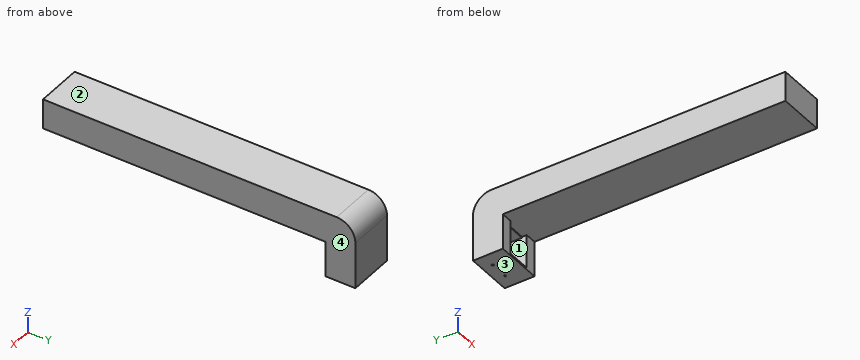
```python
from build123d import *

# Parameters (mm, degrees)
SKETCH_1_W          = 50
SKETCH_1_H          = 55
EXTRUDE_1_DEPTH     = 70
SKETCH_3_W          = 50
SKETCH_3_H          = 25
CUT_EXTRUDE_1_DEPTH = 38
SKETCH_4_W          = 25.5
SKETCH_4_H          = 36
CUT_EXTRUDE_2_DEPTH = 22
SKETCH_12_W         = 25.5
SKETCH_12_H         = 1
EXTRUDE_2_DEPTH     = 19
EXTRUDE_3_DEPTH     = 2
SKETCH_16_W         = 50
SKETCH_16_H         = 32
EXTRUDE_5_DEPTH     = 280
FILLET_1_R          = 20
SKETCH_23_R         = 1
CUT_EXTRUDE_3_DEPTH = 10


with BuildPart() as part:
    # 草图1 → 凸台-拉伸1 (new body)
    with BuildSketch(Plane.XY):
        with Locations((25, 27.5)):
            Rectangle(SKETCH_1_W, SKETCH_1_H)
    extrude(amount=EXTRUDE_1_DEPTH)

    # 草图3 → 切除-拉伸1 (cut)
    with BuildSketch(Plane(origin=(0, 0, 0), x_dir=(-1, 0, 0), z_dir=(0, 0, -1))):
        with Locations((-25, 12.5)):
            Rectangle(SKETCH_3_W, SKETCH_3_H)
    extrude(amount=-CUT_EXTRUDE_1_DEPTH, mode=Mode.SUBTRACT)

    # 草图4 → 切除-拉伸2 (cut)
    with BuildSketch(Plane.XZ.offset(-25)):
        with Locations((24.95, 20)):
            Rectangle(SKETCH_4_W, SKETCH_4_H)
    extrude(amount=-CUT_EXTRUDE_2_DEPTH, mode=Mode.SUBTRACT)

    # 草图12 → 凸台-拉伸2 (add)
    with BuildSketch(Plane.XZ.offset(-47)):
        with Locations((24.95, 37.5)):
            Rectangle(SKETCH_12_W, SKETCH_12_H)
    extrude(amount=EXTRUDE_2_DEPTH)

    # 草图13 → 凸台-拉伸3 (add)
    with BuildSketch(Plane.XZ.offset(-25)):
        Polygon((12.2, 38), (0, 38), (0, 0), (50, 0), (50, 38), (37.7, 38), (37.7, 2), (12.2, 2), align=None)
    extrude(amount=EXTRUDE_3_DEPTH)

    # 草图16 → 凸台-拉伸5 (add)
    with BuildSketch(Plane.XZ):
        with Locations((25, 54)):
            Rectangle(SKETCH_16_W, SKETCH_16_H)
    extrude(amount=EXTRUDE_5_DEPTH)

    # 圆角1
    fillet_1_edges = [part.edges().sort_by_distance(p)[0] for p in [
        (25, 55, 70),
    ]]
    fillet(fillet_1_edges, radius=FILLET_1_R)

    # 草图23 → 切除-拉伸3 (cut)
    with BuildSketch(Plane(origin=(0, 0, 0), x_dir=(-1, 0, 0), z_dir=(0, 0, -1))):
        with Locations((-15.2, 44.140200043)):
            Circle(SKETCH_23_R)
        with Locations((-34.8, 44.140200043)):
            Circle(SKETCH_23_R)
    extrude(amount=-CUT_EXTRUDE_3_DEPTH, mode=Mode.SUBTRACT)


solid = part.part
```
Could you check a few things on this model? Use its own coordinates, in mm. Face numbers are marked on the shaded views. Round coordinates to 2 decimals unless told otherwise and drop trailing zeros. Write each loop counter-clockwise with the first axis right and the second up, starting at its lowest first coordinate (ties: lowest second). Pieces come first, ordered by that corner, then holes.
(1) Thinking about a two-plate mould opening in Z: for the marked faces 1, 2, 3 and 4, which applies, +Z half, -Z half, draft (parallel to the pull), parting line (faces both ways), or undercut?
Findings below:
face 1: undercut
face 2: +Z half
face 3: -Z half
face 4: draft
(2) Suppose I cut it at D-D on x = 20.5. Write out the boundary of the cut face in (y, z).
Findings below:
outline: (-280, 38) - (28, 38) - (28, 37) - (47, 37) - (47, 2) - (23, 2) - (23, 0) - (55, 0) - (55, 50) arc R20 ccw to (35, 70) - (-280, 70) - close
(3) Suppose I cut it at A-A on z = 30.5. Write out the boundary of the cut face in (x, y).
Findings below:
outline: (0, 23) - (12.2, 23) - (12.2, 47) - (37.7, 47) - (37.7, 23) - (50, 23) - (50, 55) - (0, 55) - close
(4) For pin 1 (1.2 mm diameter, centred on x = 15.2, y = 44.14, fed in from -Z); pin 2 (8 mm diameter, centred on x = 40, y = -48, fed in from -Z); pin 3 (1 mm diameter, centred on x = 30.5, z = 13, fed in from -Y), each with a flat end and sliding along its axis, tell me the tip position at first contact or that it passes through.
Findings below:
pin 1: stops at z = 37
pin 2: stops at z = 38
pin 3: stops at y = 47
(5) Suppose I cut it at B-B on x = 7. Write out the boundary of the cut face in (y, z), and give its area (3 significant figures).
Findings below:
outline: (-280, 38) - (23, 38) - (23, 0) - (55, 0) - (55, 50) arc R20 ccw to (35, 70) - (-280, 70) - close
area: 11,900 mm2
(6) If I drill on probe 1 along X at (y, z) = (38.5, 22.5); probe 2 along Y at (x, z) = (15, 1); probe 3 along Y at (x, z) = (15.2, 0.9), over which ranges is the centre line in solid material (lowest first)?
Findings below:
probe 1: x = 0 to 12.2, 37.7 to 50
probe 2: y = 23 to 43.16, 45.12 to 55
probe 3: y = 23 to 43.14, 45.14 to 55
(7) Suppose I cut it at C-C on y = -236. Write out the boundary of the cut face in (x, z), and give its area (3 significant figures).
Findings below:
outline: (0, 38) - (50, 38) - (50, 70) - (0, 70) - close
area: 1,600 mm2
